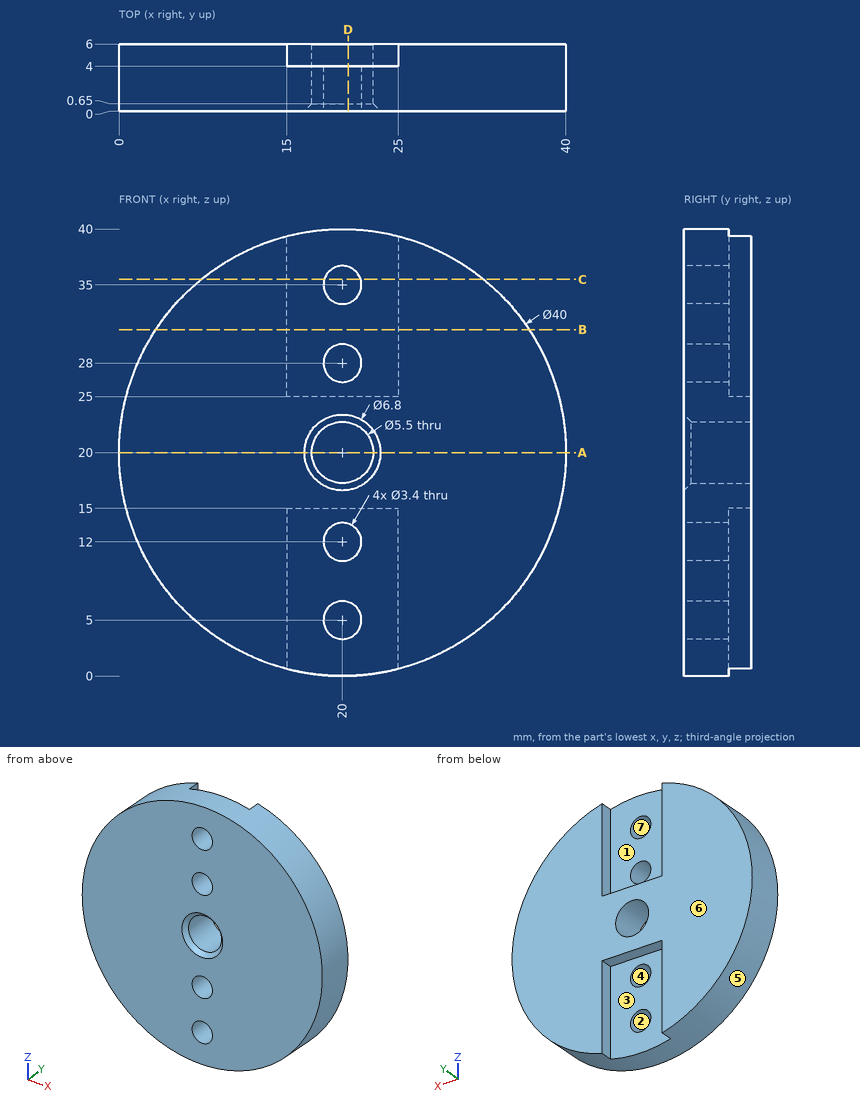
Input: dimensioned drawing with shaded views. Units: mm. Origin: part minimum x, y, z. A direction names the side the tool comes from. Give positions to 0.01 mm unless a question says otherwise; leave off trailing zeros. Loops run counter-clockwise (first coordinate to the right, second up) from the corner with the lowest first, then second, coordinate; pieces in that order, holes last. Notation, with made-up numbers: M 2.5,18.25 L 51.5,18.25 A25 cw 51.5,38.25 Z; hole C -39.75,63 d1. An arc over 180 degrees is marked long. Put each result on its own line as item: value. Start each with the question number.
1) Contact query for flat-ended pins moving along their axis: pin 1 (4 mm diameter, centred on x = 20, z = 35, fed in from +Y); pin 2 (0.6 mm diameter, centred on y = 5, z = 32.5, fed in from +X); pin 3 (2 mm diameter, centred on y = 5.5, z = 34, fed in from -X); pin 4 (2.5 mm diameter, centred on x = 20, z = 12, fed in from -Y). Output: stop coordinate, or through.
2) Cut plane B-B (z = 31). Output: boundary loops of the cut face in (x, y).
3) Cut plane C-C (z = 35.5). Output: boundary loops of the cut face in (x, y).
4) Access query for the marked faces 1, 2 and 3. Directions: +Z, -Z, +X, -X, +Y, -Y. A direction counts if a zero-diameter tool reaches every point of the face in a straight line with its end or side. Return the directions, or none.
5) Cut plane D-D (x = 20.5). Give the number of separate pieces and of enclosed holes in the cut face, then the cut area to 3 significant figures.
6) Ray query, line 1 along Z through (x, y) = (20, 2.3); line 2 along X through (y, z) = (0.8, 27) (3 decimals); line 3 along X through (y, z) = (4.45, 13) (3 decimals). Return the intervals inside material, ascending.
7) Cut plane A-A (z = 20). Output: boundary loops of the cut face in (x, y).
8) Pull-direction query (Z, two-part tool) for the marked faces 4, 5, 6 and 7; classes: pulls with the +Z half, pulls with the -Z half, needs draft (parallel to the pull), parting line crosses it, or undercut.
Verdict:
1. pin 1: y = 4
1. pin 2: x = 35.85
1. pin 3: x = 4.8
1. pin 4: through
2. outline: M 3.3,0 L 36.7,0 L 36.7,6 L 25,6 L 25,4 L 15,4 L 15,6 L 3.3,6 Z
3. outline: M 7.36,0 L 18.38,0 L 18.38,4 L 15,4 L 15,6 L 7.36,6 Z; M 21.62,0 L 32.64,0 L 32.64,6 L 25,6 L 25,4 L 21.62,4 Z
4. face 1: +Z, +Y
4. face 2: +Y, -Y
4. face 3: -Z, +Y
5. separate pieces: 6
5. enclosed holes: 0
5. area: 95.1 mm2
6. line 1: 0 to 3.3, 6.7 to 10.3, 13.7 to 17.25, 22.75 to 26.3, 29.7 to 33.3, 36.7 to 40
6. line 2: 1.265 to 18.625, 21.375 to 38.735
6. line 3: 1.265 to 15, 25 to 38.735
7. outline: M 0,0 L 16.6,0 L 17.25,0.65 L 17.25,6 L 0,6 Z; M 22.75,0.65 L 23.4,0 L 40,0 L 40,6 L 22.75,6 Z
8. face 4: undercut
8. face 5: parting line crosses it
8. face 6: needs draft
8. face 7: undercut
